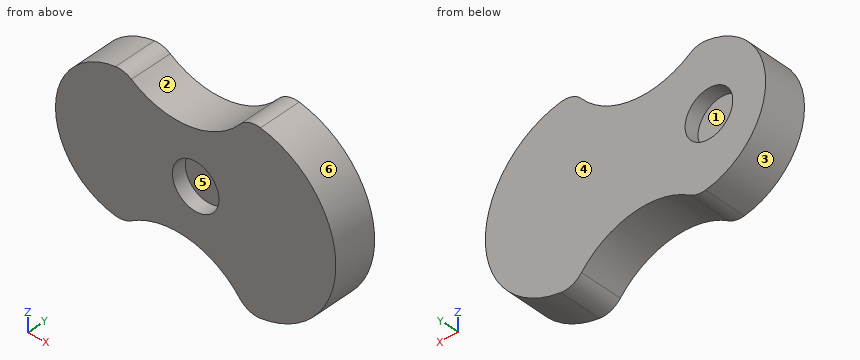
Autodesk Inventor part; units mm, degrees
ref_plane "YZ Plane" through (0, 0, 0) normal (1, 0, 0) x (0, 1, 0)
ref_plane "XZ Plane" through (0, 0, 0) normal (0, 1, 0) x (-1, 0, 0)
ref_plane "XY Plane" through (0, 0, 0) normal (0, 0, 1) x (1, 0, 0)
sketch "Sketch1" plane through (0, 0, 0) normal (0, 1, 0) x (-1, 0, 0)
  circle A0 centre (0, 0) radius 25
  dimension "d0" = 50
extrude "Extrusion1" add sketch "Sketch1" along normal blind 10
sketch "Sketch2" plane through (0, 0, 0) normal (0, -1, 0) x (1, 0, 0)
  circle A0 centre (0, 0) radius 4.15
  dimension "d3" = 8.3
extrude "Extrusion2" cut sketch "Sketch2" against normal blind 2.5
sketch "Sketch8" plane through (0, 10, 0) normal (0, 1, 0) x (1, 0, 0)
  point P0 (0, 0)
sketch "Sketch9" plane through (0, 10, 0) normal (0, 1, 0) x (1, 0, 0)
  circle A0 centre (0, 0) radius 25
  circle A1 centre (-12.5, 0) radius 12.5
  circle A2 centre (9, 0) radius 16
  arc A3 (9, -16) -> (-12.5, -12.5) centre (-3.2934, -23.7306) ccw
  arc A4 (-12.5, 12.5) -> (9, 16) centre (-3.2934, 23.7306) ccw
  point P0 (-25, 0)
  point P1 (25, 0)
  dimension "d17" = 32
extrude "Extrusion6" cut sketch "Sketch9" against normal blind 15 contours A2 A1 A0 | A0 A1 A2 | A4 A2 | A2 A3 | A1 A4 | A3 A1
fillet "Fillet3" radius 4 1 edges at (-12.5, 5, 12.5)
fillet "Fillet4" radius 4 1 edges at (9, 5, 16)
fillet "Fillet5" radius 4 1 edges at (-12.5, 5, -12.5)
fillet "Fillet6" radius 4 1 edges at (9, 5, -16)
sketch "Sketch10" plane through (0, 10, 0) normal (0, 1, 0) x (1, 0, 0)
  circle A0 centre (0, 0) radius 4.15
  circle A1 centre (0, 0) radius 29.3218
extrude "Extrusion7" cut sketch "Sketch10" against normal blind 2.5 contours A0 | A1
sketch "Sketch11" plane through (0, 7.5, 0) normal (0, 1, 0) x (1, 0, 0)
  circle A0 centre (-14.875, 0) radius 4.25
  point P0 (0, 0)
  dimension "d26" = 8.5
extrude "Extrusion8" cut sketch "Sketch11" against normal blind 2.5
properties part number "Axel"
CAD build for the part. Positions are in the model's coordinates, mm. Face numbers are marked on the shaded views. A direction names the side the tool comes from. Coordinates: 2 decimals unless noted, no trailing zeros. Order: outer loops, then holes, each group sorted by start corner. A loop starts at its lowest first (then second) coordinate and runs counter-clockwise, first axis right, second up. Notation, with made-up numbers: (23.25, 75.25) -> (33.25, 75.25) arc R17 ccw to (33.25, 99.25) -> close; hole circle Ø2 at (13.5, 83). An arc over 180 degrees is marked (long way). Answer in a Markdown table with one row per item.
1) Mould opens along X. For the marked faces 1, 2, 3 and 4 say: pulls with the +X half, pulls with the -X half, needs draft (parallel to the pull), parting line crosses it, or undercut.
Check values:
| item | result |
|---|---|
| face 1 | undercut |
| face 2 | undercut |
| face 3 | pulls with the -X half |
| face 4 | needs draft |
2) Which spindle directions (+Z, -Z, +X, -X, +Y, -Y) get a long thin tool onto all of the face, cutting with end or side? Do the marked faces 5 and 6. Say none if no direction does.
Check values:
| item | result |
|---|---|
| face 5 | -Y |
| face 6 | +X, +Y, -Y |
3) Drill centre lines: line 1 (X direction, y = 6.5, z = 0) (3 decimals); line 2 (Y direction, x = -0.5, z = 2); line 3 (X direction, y = 1.5, z = 0.5). Where is each one in solid material? Low to high.
Check values:
| item | result |
|---|---|
| line 1 | -25 to -19.125, -10.625 to 25 |
| line 2 | 2.5 to 7.5 |
| line 3 | -24.99 to -4.12, 4.12 to 24.99 |
4) Flat gauge pins, fed straight in: P1, Ø7, axis at x = -14.875, z = 0, coming from the +Y side; P2, Ø1.5, axis at x = -15, y = 4.5, coming from the +Z side; P3, Ø4, axis at x = 2, z = 0, coming from the -Y side. Where does each tip first touch, or does it go through?
Check values:
| item | result |
|---|---|
| P1 | y = 5 |
| P2 | z = 12.38 |
| P3 | y = 2.5 |
5) Band-saw the part on A-A (z = 0). List the corners of the cut face in (x, y) (3 decimals), and give its area (3 significant figures).
Check values:
| item | result |
|---|---|
| outline | (-25, 0) -> (-4.15, 0) -> (-4.15, 2.5) -> (4.15, 2.5) -> (4.15, 0) -> (25, 0) -> (25, 7.5) -> (-10.625, 7.5) -> (-10.625, 5) -> (-19.125, 5) -> (-19.125, 7.5) -> (-25, 7.5) -> close |
| area | 333 mm2 |
6) Band-saw the part on B-B (x = -18.5). List the corners of the cut face in (y, z), and give its area (3 significant figures).
Check values:
| item | result |
|---|---|
| outline | (0, -10.97) -> (7.5, -10.97) -> (7.5, -2.22) -> (5, -2.22) -> (5, 2.22) -> (7.5, 2.22) -> (7.5, 10.97) -> (0, 10.97) -> close |
| area | 153 mm2 |
7) Band-saw the part on C-C (x = -3.5). List the corners of the cut face in (y, z), and give its area (3 significant figures).
Check values:
| item | result |
|---|---|
| outline | (0, -9.21) -> (7.5, -9.21) -> (7.5, 9.21) -> (0, 9.21) -> (0, 2.23) -> (2.5, 2.23) -> (2.5, -2.23) -> (0, -2.23) -> close |
| area | 127 mm2 |
8) Band-saw the part on D-D (z = -6). List the corners of the cut face in (x, y), and give its area (3 significant figures).
Check values:
| item | result |
|---|---|
| outline | (-23.47, 0) -> (23.83, 0) -> (23.83, 7.5) -> (-23.47, 7.5) -> close |
| area | 355 mm2 |
